Autodesk Inventor part; units mm, degrees
ref_plane "Work Plane1" through (30.1625, 0, 0) normal (0, 0, -1) x (1, 0, 0)
ref_plane "YZ Plane" through (0, 0, 0) normal (1, 0, 0) x (0, 1, 0)
ref_plane "XZ Plane" through (0, 0, 0) normal (0, 1, 0) x (-1, 0, 0)
sketch "Schizzo1" plane through (0, 0, 0) normal (0, 0, 1) x (1, 0, 0)
  line L0 (-2.4, 0) -> (12, 0)
  line L1 (12, 0) -> (12, 2)
  line L2 (12, 2) -> (1.4, 2)
  line L3 (1.4, 2) -> (0.9705, 1.7853)
  line L4 (0.9705, 1.7853) -> (0, 1.7853)
  line L5 (0, 1.7853) -> (0, 4)
  line L6 (-5.28, 0) -> (14.88, 0)
  line L7 (0, -0.8) -> (0, 4.8)
  line L8 (-2.4, 0) -> (-2.4, 3.79)
  line L9 (0, 4) -> (-2.4, 3.79)
  line L10 (1.4, 2) -> (0, 2) construction
  dimension "d0" = 12
  dimension "d1" = 10.6
  dimension "d2" = 0.4295
  dimension "d3" = 2.4
  dimension "d4" = 4
  dimension "d5" = 3.5705
  dimension "d9" = 8
  dimension "d10" = 5
revolve "Corpo" add sketch "Schizzo1" angle 360 about axis through (-2.4, 0, 0) along (1, 0, 0)
sketch "Schizzo2" plane through (-2.4, 0, 0) normal (-1, 0, 0) x (0, 0, 1)
  circle A0 centre (0, 0) radius 4
  line L0 (0, 0) -> (0, 3.79)
  line L1 (-4, 0.6) -> (4, 0.6)
  line L2 (4, 0.6) -> (4, -0.6)
  line L3 (4, -0.6) -> (-4, -0.6)
  line L4 (-4, -0.6) -> (-4, 0.6)
  line L5 (-4, 0) -> (4, 0) construction
  line L6 (0, 0.6) -> (0, -0.6) construction
  dimension "d11" = 1.2
  dimension "d12" = 8
fillet "Raccordo1" radius 1.2 1 edges at (-2.4, -3.79, 0)
extrude "Intaglio" cut sketch "Schizzo2" against normal blind 1 contours A0 L3 L1 | L2 L3 A0 | A0 L1 L2 | A0 L4 L1 | L3 L4 A0
thread "Filettatura"
ref_plane "Work Plane1" through (30.1625, 0, 0) normal (0, 0, -1) x (1, 0, 0)
fillet "Fillet5" radius 0.2 1 edges at (0, -1.7853, 0)
equation "\"d11\" = SBR"
equation "\"d12\" = KOD"
equation "\"d14\" = RR"
equation "\"d19\" = STI"
equation "\"d15\" = GEL"
equation "\"d41\" = R"
equation "\"d0\" = NLG"
equation "\"d1\" = GEL"
equation "\"d3\" = KOH"
equation "\"d4\" = GD"
equation "\"d5\" = BDM"
equation "\"d9\" = KOD"
equation "\"d10\" = KEWI"
equation "\"GD\" = NND"
equation "\"NLG\" = 12"
equation "\"GEL\" = 10.6"
equation "\"KOD\" = 8"
equation "\"KOH\" = 2.4"
equation "\"GAL\" = 0.61345 * PTC"
equation "\"R\" = 0.2"
equation "\"BDM\" = 3.5705"
equation "\"GUL\" = 0.61345 * PTC"
equation "\"RR\" = 1.2"
equation "\"SBR\" = 1.2"
equation "\"STI\" = 1"
equation "\"KEWI\" = 5deg"
equation "\"PTC\" = 0.7"
equation "\"THREADDIA\" = 4"
equation "\"TOA\" = 30deg"
equation "\"NND\" = 4"
equation "\"GD1\" = THREADDIA - 1.2269 * PTC"
properties part number "ISO 1580 - M4 x 12" material "Acciaio, Dolce"
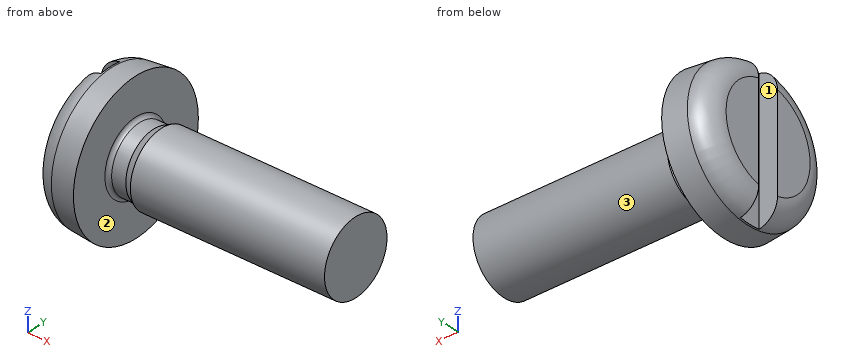
Build history of the part. All positions in model axes, mm. Face numbers are marked on the shaded views. Give positions to 0.01 mm unless a question says otherwise; leave off trailing zeros. Loops run counter-clockwise (first coordinate to the right, second up) from the corner with the lowest first, then second, coordinate; pieces in that order, holes last. Notation, with made-up numbers: (-23.5, -8.5) - (35.5, -8.5) arc R25 ccw to (35.5, 10.5) - close; hole circle Ø2 at (76, -27.5). An arc over 180 degrees is marked (long way). Write item = value, one per line. Start each with the question number.
1) Drop flat-ended pins along their axis: pin 1 Ø1 at (y, z) = (0, -0.5) entering from -X; pin 2 Ø1.5 at (x, y) = (5.5, 1.5) entering from -Z; pin 3 Ø2 at (y, z) = (3, 2.5) entering from +X. Give the stop position or say it passes through.
2) Pull direction Y, two halves, no side cores. Call the marked faces 1, 2 and 3: +Y half, -Y half, draft (parallel to the pull), parting line (faces both ways), or undercut.
3) Band-saw the part on B-B on y = 0. Give the cut face in (x, z), plus the area to 3 significant figures.
4) Probe probe 1 along X at (y, z) = (-1, -2); probe 2 along Z at (x, y) = (4.5, -0.25); probe 3 along X at (y, z) = (0.25, -0.25). List the from-to ranges inside material, lowest first. Write a range as from..to.
5) Band-saw the part on D-D on x = 1.25. Give the cut face in (y, z), plus the area to 3 significant figures.
6) Band-saw the part on C-C on x = 7.5. Give the cut face in (y, z).
7) Band-saw the part on A-A on z = 0. Give the cut face in (x, y).
Final values:
q1.pin_1 = -1.4
q1.pin_2 = -1.85
q1.pin_3 = 0
q2.face_1 = undercut
q2.face_2 = draft
q2.face_3 = parting line
q3.outline = (-1.4, -3.87) arc R1.2 ccw to (-1.3, -3.89) - (0, -4) - (0, -1.99) arc R0.2 cw to (0.2, -1.79) - (0.97, -1.79) - (1.4, -2) - (12, -2) - (12, 2) - (1.4, 2) - (0.97, 1.79) - (0.2, 1.79) arc R0.2 cw to (0, 1.99) - (0, 4) - (-1.3, 3.89) arc R1.2 ccw to (-1.4, 3.87) - close
q3.area = 58.5 mm²
q4.probe_1 = -2.4..0
q4.probe_2 = -1.98..1.98
q4.probe_3 = -1.4..12
q5.outline = circle Ø3.85 at (0, 0)
q5.area = 11.6 mm²
q6.outline = circle Ø4 at (0, 0)
q7.outline = (-2.4, -2.69) arc R1.2 ccw to (-1.3, -3.89) - (0, -4) - (0, -1.99) arc R0.2 cw to (0.2, -1.79) - (0.97, -1.79) - (1.4, -2) - (12, -2) - (12, 2) - (1.4, 2) - (0.97, 1.79) - (0.2, 1.79) arc R0.2 cw to (0, 1.99) - (0, 4) - (-1.3, 3.89) arc R1.2 ccw to (-2.4, 2.69) - (-2.4, 0.6) - (-1.4, 0.6) - (-1.4, -0.6) - (-2.4, -0.6) - close
